Autodesk Fusion 360 part; units mm, degrees
sketch "Sketch1" plane through (0, 0, 0) normal (0, 0, 1) x (1, 0, 0)
  circle A0 centre (0, 0) radius 16
  circle A1 centre (0, 0) radius 13 construction
  line L0 (0, 0) -> (0, 16) construction
  circle A2 centre (0, 13) radius 2
  circle A3 centre (-13, 0) radius 2
  circle A4 centre (0, -13) radius 2
  circle A5 centre (13, 0) radius 2
  circle A6 centre (0, 0) radius 6
  dimension "d1" = 32
  dimension "d2" = 26
  dimension "d3" = 4
  dimension "d5" = 360
  dimension "d6" = 12
extrude "Extrude1" add sketch "Sketch1" along normal blind 3
sketch "Sketch2" plane through (0, 0, 3) normal (0, 0, 1) x (-1, 0, 0)
  circle A0 centre (0, -13) radius 2
  circle A1 centre (13, 0) radius 2
  circle A2 centre (0, 13) radius 2
  circle A3 centre (-13, 0) radius 2
  circle A4 centre (0, 0) radius 6
  circle A5 centre (0, 0) radius 16
  circle A6 centre (0, 0) radius 9
  dimension "d9" = 18
extrude "Extrude2" add sketch "Sketch2" along normal blind 10 contours A6
ref_plane "WorkPlane1" through (6.364, -6.364, 9.993) normal (0.7071, -0.7071, 0) x (-0.7071, -0.7071, 0)
sketch "Sketch3" plane through (6.364, -6.364, 0) normal (0.7071, -0.7071, 0) x (-0.7071, -0.7071, 0)
  line L0 (-9, -13) -> (9, -13) construction
  line L1 (9, -3) -> (-9, -3) construction
  line L2 (0, -13) -> (0, -3) construction
  circle A0 centre (0, -8) radius 2
  line L3 (0, -8) -> (0, -10) construction
  dimension "d13" = 4
  dimension "d14" = 3
extrude "Extrude3" cut sketch "Sketch3" against normal blind 20
Geometry check sheet. Reference: the model listing, model coordinates, mm. A direction names the side the tool comes from. Round coordinates to 2 decimals unless told otherwise and drop trailing zeros. Loops run counter-clockwise (first coordinate to the right, second up) from the corner with the lowest first, then second, coordinate; pieces in that order, holes last.
Item 1: Gauge pin test, flat ends, axial feed: pin 1 (9.5 mm diameter, centred on x = 0, y = 0, fed in from +Z); pin 2 (1.5 mm diameter, centred on y = 2, z = 10.5, fed in from +X); pin 3 (4 mm diameter, centred on y = -7, z = 1.5, fed in from -X); pin 4 (6 mm diameter, centred on y = 0.5, z = 9, fed in from -X). Record the tip position at first contact, or that the pin passes through.
Item 2: Cross-section at D-D on z = 1.5. Record the boundary of the cut face in (x, y).
Item 3: Cross-section at B-B on y = -12. Record the boundary of the cut face in (x, z).
Item 4: Access from +Z, -Z, +X, -X, +Y, -Y to the whole of each face (thin tool, end or side, straight path). Record for faces 1 (the cylindrical face through (0, 6, 6)), 2 (the flat face through (7, -7, 3)).
Item 5: Cross-section at C-C on z = 7.25. Record the boundary of the cut face in (x, y).
Item 6: Mould release check, pull along X, two halves, no side actions. Record for faces 3 (the cylindrical face through (11.4, 1.2, 1.5)), 4 (the flat face through (-2, 6, 13)), 5 (the cylindrical face through (-8.584, 2.703, 7.93)): pulls with the +X half, pulls with the -X half, needs draft (parallel to the pull), parting line crosses it, or undercut.
Item 7: Thickness scan on line 1 (X direction, y = -1, z = 1.75); line 2 (Y direction, x = -0.5, z = 1.25); line 3 (Z direction, x = 11, y = -7). Record the ranges inside material, lowest first.
Answer sheet:
1. pin 1: passes through
1. pin 2: stops at x = 8.91
1. pin 3: stops at x = -15.2
1. pin 4: stops at x = -9
2. outline: circle Ø32 at (0, 0); hole circle Ø4 at (-13, 0); hole circle Ø12 at (0, 0); hole circle Ø4 at (0, -13); hole circle Ø4 at (0, 13); hole circle Ø4 at (13, 0)
3. outline: (-10.58, 0) - (-1.73, 0) - (-1.73, 3) - (-10.58, 3) - close; (1.73, 0) - (10.58, 0) - (10.58, 3) - (1.73, 3) - close
4. face 1: +Z, -Z
4. face 2: +Z
5. outline: (-7.54, 4.92) arc R9 ccw to (4.92, -7.54) - (2.72, -5.35) arc R6 cw to (-5.35, 2.72) - close; (-4.92, 7.54) - (-2.72, 5.35) arc R6 cw to (5.35, -2.72) - (7.54, -4.92) arc R9 ccw to start
6. face 3: undercut
6. face 4: needs draft
6. face 5: parting line crosses it
7. line 1: x = -15.97 to -14.73, -11.27 to -5.92, 5.92 to 11.27, 14.73 to 15.97
7. line 2: y = -15.99 to -14.94, -11.06 to -5.98, 5.98 to 11.06, 14.94 to 15.99
7. line 3: z = 0 to 3
